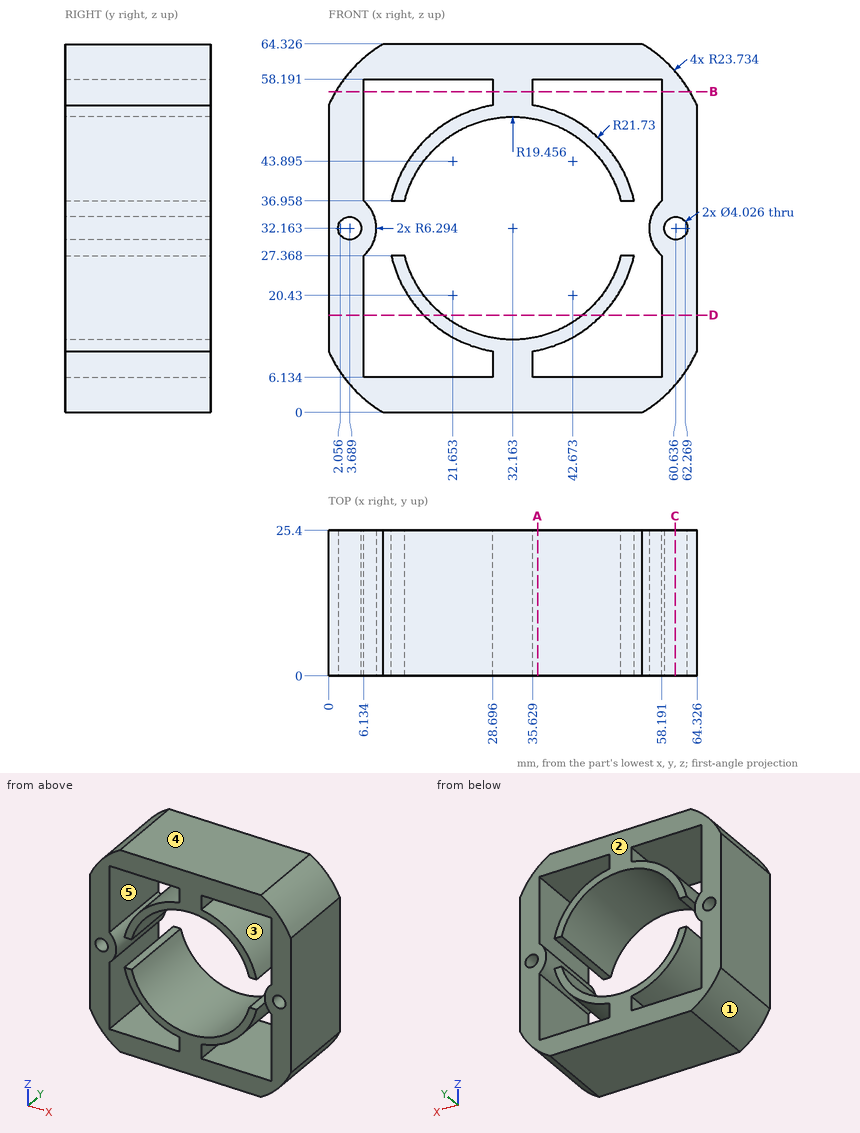
Design review of the part shown in the three views and the two pictorial views. Dimensions are in mm from the part's minimum x, y and z. A direction names the side the tool comes from. Give positions to 0.01 mm unless a question says otherwise; leave off trailing zeros. Loops run counter-clockwise (first coordinate to the right, second up) from the corner with the lowest first, then second, coordinate; pieces in that order, holes last. Notation, with made-up numbers: M 24.5,65.5 L 52.5,65.5 A21 cw 52.5,96.5 Z; hole C 61.5,62.5 d7. An arc over 180 degrees is marked long. Put each result on its own line as item: value. Start each with the question number.
(1) Add section D-D, the plane z = 17. Write out the cut boundary in (x, y) (1 decimal), then the cut area to 3 significant figures.
(2) For pin 1 (1 mm diameter, centred on y = 13.5, z = 10.5, fed in from +X) (1 decimal); pin 2 (3 mm diameter, centred on x = 3.69, z = 32.16, fed in from -Y); pin 3 (5 mm diameter, centred on y = 12, z = 57, fed in from +X) (1 decimal), all flat-tipped, find the tip position at first contact; note any pin that passes through.
(3) Machinability: for the marked faces 4 and 5, which of the approach directions +Z, -Z, +X, -X, +Y, -Y give a long, thin tool a straight path to every point of the face, cutting with its end or side? Answer none if there is none.
(4) Add section B-B, the plane z = 56. Write out the cut boundary in (x, y) (1 decimal).
(5) Add section C-C, the plane x = 60.5. Write out the cut boundary in (y, z) (1 decimal), then the cut area to 3 significant figures.
(6) Wall thickness on L1, parallel to X at y = 13.25, z = 32 (1 decimal); L2, parallel to X at y = 6.75, z = 17 (1 decimal): over which ranges is each line inside the solid? List them lowest first.
(7) Add section A-A, the plane x = 36.5. Write out the cut boundary in (y, z) (1 decimal).
(8) The part is to be moulded in two halves that separate along Z. For the marked faces 1, 2 and 3, say which applies: +Z half, -Z half, draft (parallel to the pull), parting line (faces both ways), or undercut.
Result:
1. outline: M 0,0 L 6.1,0 L 6.1,25.4 L 0,25.4 Z; M 16.6,0 L 20,0 L 20,25.4 L 16.6,25.4 Z; M 44.4,0 L 47.7,0 L 47.7,25.4 L 44.4,25.4 Z; M 58.2,0 L 64.3,0 L 64.3,25.4 L 58.2,25.4 Z
1. area: 483 mm^2
2. pin 1: stops at x = 64.3
2. pin 2: passes through
2. pin 3: stops at x = 63.9
3. face 4: +Z, +X, -X, +Y, -Y
3. face 5: +Y, -Y
4. outline: M 1.2,0 L 6.1,0 L 6.1,25.4 L 1.2,25.4 Z; M 28.7,0 L 35.6,0 L 35.6,25.4 L 28.7,25.4 Z; M 58.2,0 L 63.1,0 L 63.1,25.4 L 58.2,25.4 Z
5. outline: M 0,4.8 L 25.4,4.8 L 25.4,30.2 L 0,30.2 Z; M 0,34.2 L 25.4,34.2 L 25.4,59.6 L 0,59.6 Z
5. area: 1,290 mm^2
6. L1: x = 0 to 1.7, 5.7 to 8.3, 56 to 58.6, 62.6 to 64.3
6. L2: x = 0 to 6.1, 16.6 to 20, 44.4 to 47.7, 58.2 to 64.3
7. outline: M 0,0 L 25.4,0 L 25.4,6.1 L 0,6.1 Z; M 0,10.9 L 25.4,10.9 L 25.4,13.2 L 0,13.2 Z; M 0,51.1 L 25.4,51.1 L 25.4,53.5 L 0,53.5 Z; M 0,58.2 L 25.4,58.2 L 25.4,64.3 L 0,64.3 Z
8. face 1: -Z half
8. face 2: draft
8. face 3: undercut
